from build123d import *

# Parameters (mm, degrees)
F0_R     = 1.5875
F0_R_2   = 22.225
F1_DEPTH = 2.9972
F2_DEPTH = 25.4
F3_DEPTH = 25.4
F4_DEPTH = 12.7
F5_DEPTH = 2.9972
F6_DEPTH = 5.9944


# Not quite as in the source:
# - a fillet or chamfer that OpenCascade refuses, or shapes differently, is made with other operations: its cross-section is extruded or revolved along the edge and cut away or added


with BuildPart() as f1:
    # F0 (on Top) → F1 (new body)
    with BuildSketch(Plane.XY):
        with BuildLine():
            Line((-78.3343552322, -16.2264228234), (-86.7801633577, -25.6357348999))
            ThreePointArc((-86.7801633577, -25.6357348999), (-83.5995491981, -34.6280670861), (-79.4900439712, -43.2356399943))
            Line((-79.4900439712, -43.2356399943), (-66.8645673974, -43.9169401718))
            ThreePointArc((-66.8645673974, -43.9169401718), (-56.5666333066, -56.5666333066), (-43.9169401718, -66.8645673974))
            Line((-43.9169401718, -66.8645673974), (-43.2356399943, -79.4900439712))
            ThreePointArc((-43.2356399943, -79.4900439712), (-34.6280670861, -83.5995491981), (-25.6357348999, -86.7801633577))
            Line((-25.6357348999, -86.7801633577), (-16.2264228234, -78.3343552322))
            ThreePointArc((-16.2264228234, -78.3343552322), (0, -79.9973), (16.2264228234, -78.3343552322))
            Line((16.2264228234, -78.3343552322), (25.6357348999, -86.7801633577))
            ThreePointArc((25.6357348999, -86.7801633577), (34.6280670861, -83.5995491981), (43.2356399943, -79.4900439712))
            Line((43.2356399943, -79.4900439712), (43.9169401718, -66.8645673974))
            ThreePointArc((43.9169401718, -66.8645673974), (56.5666333066, -56.5666333066), (66.8645673974, -43.9169401718))
            Line((66.8645673974, -43.9169401718), (79.4900439712, -43.2356399943))
            ThreePointArc((79.4900439712, -43.2356399943), (83.5995491981, -34.6280670861), (86.7801633577, -25.6357348999))
            Line((86.7801633577, -25.6357348999), (78.3343552322, -16.2264228234))
            Line((78.3343552322, -16.2264228234), (-78.3343552322, -16.2264228234))
        make_face()
        with Locations((-30.6136413439, -73.9078681262)):
            Circle(F0_R, mode=Mode.SUBTRACT)
        with Locations((30.6136413439, -73.9078681262)):
            Circle(F0_R, mode=Mode.SUBTRACT)
        with Locations((0, -47.218952328)):
            Circle(F0_R_2, mode=Mode.SUBTRACT)
        with Locations((-73.9078681262, -30.6136413439)):
            Circle(F0_R, mode=Mode.SUBTRACT)
        with Locations((73.9078681262, -30.6136413439)):
            Circle(F0_R, mode=Mode.SUBTRACT)
        with Locations((0, -47.218952328)):
            Circle(F0_R_2)
        with BuildLine():
            ThreePointArc((5.08, -32.8505425343), (12.4434078933, -38.4201342255), (15.24, -47.218952328))
            ThreePointArc((15.24, -47.218952328), (-8.7988181024, -59.6623602213), (-5.08, -32.8505425343))
            Line((-5.08, -32.8505425343), (-5.08, -26.0933935642))
            Line((-5.08, -26.0933935642), (-2.54, -26.0933935642))
            Line((-2.54, -26.0933935642), (-2.54, -32.1921096789))
            ThreePointArc((-2.54, -32.1921096789), (0, -31.978952328), (2.54, -32.1921096789))
            Line((2.54, -32.1921096789), (2.54, -26.0933935642))
            Line((2.54, -26.0933935642), (5.08, -26.0933935642))
            Line((5.08, -26.0933935642), (5.08, -32.8505425343))
        make_face(mode=Mode.SUBTRACT)
        with BuildLine():
            ThreePointArc((-5.08, -32.8505425343), (-8.7988181024, -59.6623602213), (15.24, -47.218952328))
            ThreePointArc((15.24, -47.218952328), (12.4434078933, -38.4201342255), (5.08, -32.8505425343))
            ThreePointArc((5.08, -32.8505425343), (3.8241970996, -32.466558741), (2.54, -32.1921096789))
            Line((2.54, -32.1921096789), (2.54, -34.9700344064))
            ThreePointArc((2.54, -34.9700344064), (9.7021059634, -39.3223245588), (12.5095, -47.218952328))
            ThreePointArc((12.5095, -47.218952328), (-7.8966277692, -56.9210582914), (-2.54, -34.9700344064))
            Line((-2.54, -34.9700344064), (-2.54, -32.1921096789))
            ThreePointArc((-2.54, -32.1921096789), (-3.8241970996, -32.466558741), (-5.08, -32.8505425343))
        make_face()
        with BuildLine():
            ThreePointArc((2.54, -32.1921096789), (3.8241970996, -32.466558741), (5.08, -32.8505425343))
            Line((5.08, -32.8505425343), (5.08, -26.0933935642))
            Line((5.08, -26.0933935642), (2.54, -26.0933935642))
            Line((2.54, -26.0933935642), (2.54, -32.1921096789))
        make_face()
        with BuildLine():
            Line((-5.08, -26.0933935642), (-5.08, -32.8505425343))
            ThreePointArc((-5.08, -32.8505425343), (-3.8241970996, -32.466558741), (-2.54, -32.1921096789))
            Line((-2.54, -32.1921096789), (-2.54, -26.0933935642))
            Line((-2.54, -26.0933935642), (-5.08, -26.0933935642))
        make_face()
        with BuildLine():
            Line((2.54, -34.9700344064), (2.54, -32.1921096789))
            ThreePointArc((2.54, -32.1921096789), (0, -31.978952328), (-2.54, -32.1921096789))
            Line((-2.54, -32.1921096789), (-2.54, -34.9700344064))
            ThreePointArc((-2.54, -34.9700344064), (0, -34.709452328), (2.54, -34.9700344064))
        make_face()
        with BuildLine():
            ThreePointArc((12.5095, -47.218952328), (9.7021059634, -39.3223245588), (2.54, -34.9700344064))
            ThreePointArc((2.54, -34.9700344064), (0, -34.709452328), (-2.54, -34.9700344064))
            ThreePointArc((-2.54, -34.9700344064), (-7.8966277692, -56.9210582914), (12.5095, -47.218952328))
        make_face()
    extrude(amount=F1_DEPTH)

    # F0 (on Top) → F2 (join)
    with BuildSketch(Plane.XY):
        with BuildLine():
            ThreePointArc((-5.08, -32.8505425343), (-8.7988181024, -59.6623602213), (15.24, -47.218952328))
            ThreePointArc((15.24, -47.218952328), (12.4434078933, -38.4201342255), (5.08, -32.8505425343))
            ThreePointArc((5.08, -32.8505425343), (3.8241970996, -32.466558741), (2.54, -32.1921096789))
            Line((2.54, -32.1921096789), (2.54, -34.9700344064))
            ThreePointArc((2.54, -34.9700344064), (9.7021059634, -39.3223245588), (12.5095, -47.218952328))
            ThreePointArc((12.5095, -47.218952328), (-7.8966277692, -56.9210582914), (-2.54, -34.9700344064))
            Line((-2.54, -34.9700344064), (-2.54, -32.1921096789))
            ThreePointArc((-2.54, -32.1921096789), (-3.8241970996, -32.466558741), (-5.08, -32.8505425343))
        make_face()
    extrude(amount=F2_DEPTH)

    # F0 (on Top) → F3 (join)
    with BuildSketch(Plane.XY):
        with BuildLine():
            ThreePointArc((-5.08, -32.8505425343), (-8.7988181024, -59.6623602213), (15.24, -47.218952328))
            ThreePointArc((15.24, -47.218952328), (12.4434078933, -38.4201342255), (5.08, -32.8505425343))
            ThreePointArc((5.08, -32.8505425343), (3.8241970996, -32.466558741), (2.54, -32.1921096789))
            Line((2.54, -32.1921096789), (2.54, -34.9700344064))
            ThreePointArc((2.54, -34.9700344064), (9.7021059634, -39.3223245588), (12.5095, -47.218952328))
            ThreePointArc((12.5095, -47.218952328), (-7.8966277692, -56.9210582914), (-2.54, -34.9700344064))
            Line((-2.54, -34.9700344064), (-2.54, -32.1921096789))
            ThreePointArc((-2.54, -32.1921096789), (-3.8241970996, -32.466558741), (-5.08, -32.8505425343))
        make_face()
        with BuildLine():
            ThreePointArc((2.54, -32.1921096789), (3.8241970996, -32.466558741), (5.08, -32.8505425343))
            Line((5.08, -32.8505425343), (5.08, -26.0933935642))
            Line((5.08, -26.0933935642), (2.54, -26.0933935642))
            Line((2.54, -26.0933935642), (2.54, -32.1921096789))
        make_face()
        with BuildLine():
            Line((-5.08, -26.0933935642), (-5.08, -32.8505425343))
            ThreePointArc((-5.08, -32.8505425343), (-3.8241970996, -32.466558741), (-2.54, -32.1921096789))
            Line((-2.54, -32.1921096789), (-2.54, -26.0933935642))
            Line((-2.54, -26.0933935642), (-5.08, -26.0933935642))
        make_face()
    extrude(amount=F3_DEPTH)

    # F0 (on Top) → F4 (cut)
    with BuildSketch(Plane.XY):
        with BuildLine():
            ThreePointArc((2.54, -32.1921096789), (3.8241970996, -32.466558741), (5.08, -32.8505425343))
            Line((5.08, -32.8505425343), (5.08, -26.0933935642))
            Line((5.08, -26.0933935642), (2.54, -26.0933935642))
            Line((2.54, -26.0933935642), (2.54, -32.1921096789))
        make_face()
        with BuildLine():
            Line((-5.08, -26.0933935642), (-5.08, -32.8505425343))
            ThreePointArc((-5.08, -32.8505425343), (-3.8241970996, -32.466558741), (-2.54, -32.1921096789))
            Line((-2.54, -32.1921096789), (-2.54, -26.0933935642))
            Line((-2.54, -26.0933935642), (-5.08, -26.0933935642))
        make_face()
    extrude(amount=F4_DEPTH, mode=Mode.SUBTRACT)

    # F0 (on Top) → F5 (join)
    with BuildSketch(Plane.XY):
        with BuildLine():
            ThreePointArc((2.54, -32.1921096789), (3.8241970996, -32.466558741), (5.08, -32.8505425343))
            Line((5.08, -32.8505425343), (5.08, -26.0933935642))
            Line((5.08, -26.0933935642), (2.54, -26.0933935642))
            Line((2.54, -26.0933935642), (2.54, -32.1921096789))
        make_face()
        with BuildLine():
            Line((-5.08, -26.0933935642), (-5.08, -32.8505425343))
            ThreePointArc((-5.08, -32.8505425343), (-3.8241970996, -32.466558741), (-2.54, -32.1921096789))
            Line((-2.54, -32.1921096789), (-2.54, -26.0933935642))
            Line((-2.54, -26.0933935642), (-5.08, -26.0933935642))
        make_face()
    extrude(amount=F5_DEPTH)

    # F0 (on Top) → F6 (join)
    with BuildSketch(Plane.XY):
        with Locations((0, -47.218952328)):
            Circle(F0_R_2)
        with BuildLine():
            ThreePointArc((5.08, -32.8505425343), (12.4434078933, -38.4201342255), (15.24, -47.218952328))
            ThreePointArc((15.24, -47.218952328), (-8.7988181024, -59.6623602213), (-5.08, -32.8505425343))
            Line((-5.08, -32.8505425343), (-5.08, -26.0933935642))
            Line((-5.08, -26.0933935642), (-2.54, -26.0933935642))
            Line((-2.54, -26.0933935642), (-2.54, -32.1921096789))
            ThreePointArc((-2.54, -32.1921096789), (0, -31.978952328), (2.54, -32.1921096789))
            Line((2.54, -32.1921096789), (2.54, -26.0933935642))
            Line((2.54, -26.0933935642), (5.08, -26.0933935642))
            Line((5.08, -26.0933935642), (5.08, -32.8505425343))
        make_face(mode=Mode.SUBTRACT)
        with BuildLine():
            ThreePointArc((2.54, -32.1921096789), (3.8241970996, -32.466558741), (5.08, -32.8505425343))
            Line((5.08, -32.8505425343), (5.08, -26.0933935642))
            Line((5.08, -26.0933935642), (2.54, -26.0933935642))
            Line((2.54, -26.0933935642), (2.54, -32.1921096789))
        make_face()
        with BuildLine():
            Line((-5.08, -26.0933935642), (-5.08, -32.8505425343))
            ThreePointArc((-5.08, -32.8505425343), (-3.8241970996, -32.466558741), (-2.54, -32.1921096789))
            Line((-2.54, -32.1921096789), (-2.54, -26.0933935642))
            Line((-2.54, -26.0933935642), (-5.08, -26.0933935642))
        make_face()
    extrude(amount=F6_DEPTH)

    # F7: chamfer of 6.858 x 3.1496 on 1 edges, made by hand


with BuildPart() as f7_tool2:
    # F7_s3 → F7_t4 (revolve)
    with BuildSketch(Plane.XZ.offset(47.218952328)):
        Polygon((22.225, 2.8448), (15.367, 5.9944), (22.225, 5.9944), align=None)
    revolve(axis=Axis((0, -47.218952328, 5.9944), (0, 0, 1)))

    split(bisect_by=Plane.XY.offset(2.9972), keep=Keep.TOP)


with BuildPart() as f1_1:
    add(f1.part)

    # F7_t1: cut F7_tool2
    add(f7_tool2.part, mode=Mode.SUBTRACT)


solid = f1_1.part
Here's how the part is built. I have some questions about the finished solid (model axes, mm). A direction names the side the tool comes from. Round coordinates to 2 decimals unless told otherwise and drop trailing zeros. Write each loop counter-clockwise with the first axis right and the second up, starting at its lowest first coordinate (ties: lowest second). Pieces come first, ordered by that corner, then holes.
1. For faces 1 (the flat face through (-21, -82.62, 1.48)), 2 (the flat face through (-20, -35, 2.997)), 3 (the flat face through (5.08, -30, 19)), which set-ups out of +Z, -Z, +X, -X, +Y, -Y let a thin tool reach every point of the face, with its end or its side?
2. If we mould it in two halves opening along X, with no side actions, what happens to faces 4 (the cylindrical face through (-0.04, -31.98, 4.47)), 5 (the flat face through (0, -46, 2.997)), 6 (the flat face through (-73.27, -43.57, 1.48)), 7 (the flat face through (1, -16.226, 1))? For each: released by +X, released by -X, zero draft, split by the parting line, or undercut.
3. Suppose I cut it at A-A (z = 15.5). List the corners of the cut face in (x, y) for me, and give its area (3 significant figures).
4. I need wall thicknesses on L1, parallel to Z at x = -60.5, y = -51; L2, parallel to X at y = -46.5, z = 19.75; L3, parallel to X at y = -28, z = 20.75. Which ranges of each line are inside material? Lowest first, please.
5. Suppose I cut it at B-B (x = 0). List the corners of the cut face in (y, z) for me.
6. Suppose I cut it at C-C (x = -54). List the corners of the cut face in (y, z) for me.
7. Will these pins go through, and if not, where does the flat tip stop? pin 1 Ø5 at (x, y) = (73.91, -30.61) entering from -Z; pin 2 Ø4 at (y, z) = (-54.5, 6) entering from +X; pin 3 Ø7 at (y, z) = (-32, 12.5) entering from -X; pin 4 Ø5.5 at (y, z) = (-29.5, 22) entering from -X.
Answer sheet:
1. face 1: +Z, -Z, -Y
1. face 2: +Z
1. face 3: +Z, +X, +Y
2. face 4: undercut
2. face 5: undercut
2. face 6: released by -X
2. face 7: zero draft
3. outline: (-5.08, -32.85) arc R15.24 ccw (long way) to (5.08, -32.85) - (5.08, -26.09) - (2.54, -26.09) - (2.54, -34.97) arc R12.51 cw (long way) to (-2.54, -34.97) - (-2.54, -26.09) - (-5.08, -26.09) - close
3. area: 257 mm2
4. L1: z = 0 to 3
4. L2: x = -15.22 to -12.49, 12.49 to 15.22
4. L3: x = -5.08 to -2.54, 2.54 to 5.08
5. outline: (-80, 0) - (-16.23, 0) - (-16.23, 3) - (-25.33, 3) - (-31.85, 5.99) - (-31.98, 5.99) - (-31.98, 3) - (-59.73, 3) - (-59.73, 25.4) - (-62.46, 25.4) - (-62.46, 5.99) - (-62.59, 5.99) - (-69.11, 3) - (-80, 3) - close
6. outline: (-59.02, 0) - (-16.23, 0) - (-16.23, 3) - (-59.02, 3) - close
7. pin 1: stops at z = 0
7. pin 2: stops at x = 18.38
7. pin 3: stops at x = -9.74
7. pin 4: stops at x = -5.08
